```python
from build123d import *

# Parameters (mm, degrees)
SKETCH8_R          = 40
CUT_EXTRUDE3_DEPTH = 40


with BuildPart() as part:
    # Sketch2 → Revolve4 (revolve)
    with BuildSketch(Plane.XY, mode=Mode.PRIVATE) as revolve4_sk:
        Polygon((40, 50), (40, 80), (60, 80), (60, 50), (80, 50), (80, 40), (100, 40), (100, 30), (120, 30), (120, 20), (140, 20), (140, 10), (160, 10), (160, 2.5), (180, 2.5), (180, 0), (0, 0), (0, 50), align=None)
    revolve(revolve4_sk.sketch.rotate(Axis((-106.966820462, 0, 0), (1, 0, 0)), 90), axis=Axis((-106.966820462, 0, 0), (1, 0, 0)))  # turned: the seam where the file's is

    # Sketch8 → Cut-Extrude3 (cut)
    with BuildSketch(Plane.ZY):
        Circle(SKETCH8_R)
    extrude(amount=-CUT_EXTRUDE3_DEPTH, mode=Mode.SUBTRACT)


solid = part.part
```
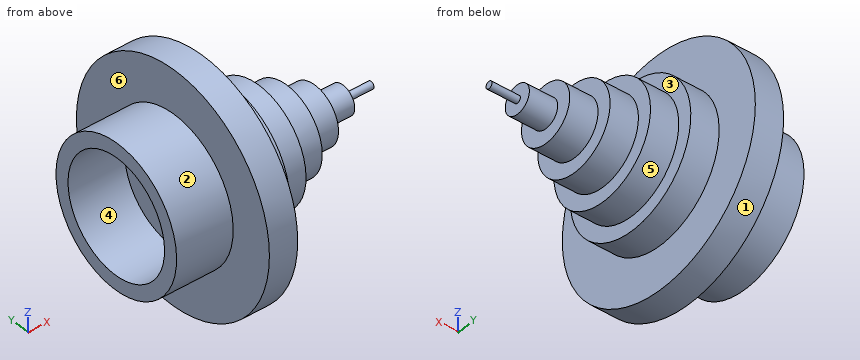
Verification items for the finished model (mm, model axes). Face numbers are marked on the shaded views. A direction names the side the tool comes from. Give positions to 0.01 mm unless a question says otherwise; leave off trailing zeros. Order: outer loops, then holes, each group sorted by start corner. A loop starts at its lowest first (then second) coordinate and runs counter-clockwise, first axis right, second up. Notation, with made-up numbers: (23, -1) - (45, -1) arc R10 ccw to (45, 16) - close; hole circle Ø3 at (-3, -3.5). An arc over 180 degrees is marked (long way). Answer as CSV lines item,"result". Start each with the question number.
Item 1: Mould release check, pull along Z, two halves, no side actions. Record for the marked faces 4, 5 and 6: released by +Z, released by -Z, zero draft, split by the parting line, or undercut.
Item 2: Access from +Z, -Z, +X, -X, +Y, -Y to the whole of each face (thin tool, end or side, straight path). Record for the marked faces 1, 2 and 3.
Item 3: Material ranges on L1, parallel to Y at x = 24.5, z = 0; L2, parallel to X at y = 66.5, z = -19.5; L3, parallel to Y at x = 113.5, z = 1, recorded low to high.
Item 4: Section check B-B, the plane x = 15.5. Record the boundary of the cut face in (y, z).
Item 5: Gauge pin test, flat ends, axial feed: pin 1 (10 mm diameter, centred on x = 83.5, y = -32.5, fed in from -Z); pin 2 (8 mm diameter, centred on x = 66, y = -25.5, fed in from -Z); pin 3 (1 mm diameter, centred on x = 56, y = -58, fed in from +Z). Record the tip position at first contact, or that the pin passes through.
Item 6: Section check D-D, the plane x = 150. Record the boundary of the cut face in (y, z), plus the area to 3 significant figures.
Item 7: Section check C-C, the plane z = 27.5. Record the boundary of the cut face in (x, y), plus the area to 3 significant figures.
Item 8: Section check A-A, the plane y = 36.5. Record the boundary of the cut face in (x, z).
Filled in:
1,face 4,"undercut"
1,face 5,"split by the parting line"
1,face 6,"zero draft"
2,face 1,"+X, -X"
2,face 2,"-X"
2,face 3,"+X"
3,L1,"-50 to -40, 40 to 50"
3,L2,"40 to 60"
3,L3,"-29.98 to 29.98"
4,outline,"circle Ø100 at (0, 0); hole circle Ø80 at (0, 0)"
5,pin 1,"z = -40.78"
5,pin 2,"z = -45.14"
5,pin 3,"z = 55.62"
6,outline,"circle Ø20 at (0, 0)"
6,area,"314 mm^2"
7,outline,"(0, -41.76) - (40, -41.76) - (40, -75.12) - (60, -75.12) - (60, -41.76) - (80, -41.76) - (80, -29.05) - (100, -29.05) - (100, -11.99) - (120, -11.99) - (120, 11.99) - (100, 11.99) - (100, 29.05) - (80, 29.05) - (80, 41.76) - (60, 41.76) - (60, 75.12) - (40, 75.12) - (40, 41.76) - (0, 41.76) - (0, 29.05) - (40, 29.05) - (40, -29.05) - (0, -29.05) - close"
7,area,"7,330 mm^2"
8,outline,"(0, -34.17) - (40, -34.17) - (40, -71.19) - (60, -71.19) - (60, -34.17) - (80, -34.17) - (80, -16.36) - (100, -16.36) - (100, 16.36) - (80, 16.36) - (80, 34.17) - (60, 34.17) - (60, 71.19) - (40, 71.19) - (40, 34.17) - (0, 34.17) - (0, 16.36) - (40, 16.36) - (40, -16.36) - (0, -16.36) - close"
